```python
from build123d import *

# Parameters (mm, degrees)
SKETCH1_R               = 10
BOSS_EXTRUDE1_DEPTH     = 15
SKETCH2_R               = 12.5
BOSS_EXTRUDE2_DEPTH     = 20
SKETCH3_R               = 12
BOSS_EXTRUDE3_DEPTH     = 139.2
SKETCH4_R               = 4.5
CUT_EXTRUDE1_DEPTH      = 176.094660113
CUT_EXTRUDE2_DEPTH      = 176.094660212
CUT_EXTRUDE2_DEPTH_BACK = 176.094660212
SKETCH5_W               = 50.129657838
SKETCH5_H               = 19.874218845
LPATTERN1_COUNT         = 2
LPATTERN1_PITCH         = 25
CUT_EXTRUDE3_DEPTH      = 176.094660212
CUT_EXTRUDE3_DEPTH_BACK = 176.094660212
SKETCH6_W               = 35.820903931
SKETCH6_H               = 2.5


with BuildPart() as part:
    # Sketch1 → Boss-Extrude1 (new body)
    with BuildSketch(Plane.XY):
        Circle(SKETCH1_R)
    extrude(amount=BOSS_EXTRUDE1_DEPTH)

    # Sketch2 → Boss-Extrude2 (add)
    with BuildSketch(Plane.XY.offset(15)):
        Circle(SKETCH2_R)
    extrude(amount=BOSS_EXTRUDE2_DEPTH)

    # Sketch3 → Boss-Extrude3 (add)
    with BuildSketch(Plane.XY.offset(35)):
        Circle(SKETCH3_R)
    extrude(amount=BOSS_EXTRUDE3_DEPTH)

    # Sketch4 → Cut-Extrude1 (cut, symmetric)
    with BuildSketch(Plane(origin=(0, 0, 0), x_dir=(1, 0, 0), z_dir=(0, 1, 0))):
        with Locations(Location((0, -154.2, 0), (0, 0, 270))):
            Circle(SKETCH4_R)
    cut_extrude1 = extrude(amount=CUT_EXTRUDE1_DEPTH, both=True, mode=Mode.SUBTRACT)

    # Sketch5 → Cut-Extrude2 (cut, two sides: drawn at the far end of the back side and taken through both)
    with BuildSketch(Plane(origin=(0, 0, 0), x_dir=(1, 0, 0), z_dir=(0, 1, 0)).offset(-CUT_EXTRUDE2_DEPTH_BACK)):
        with Locations((-12.564828919, -5.062890578)):
            Rectangle(SKETCH5_W, SKETCH5_H)
    extrude(amount=CUT_EXTRUDE2_DEPTH + CUT_EXTRUDE2_DEPTH_BACK, mode=Mode.SUBTRACT)

    # LPattern1: Cut-Extrude1 ×2
    with Locations(*[(0, 0, -i * LPATTERN1_PITCH) for i in range(1, LPATTERN1_COUNT)]):
        add(cut_extrude1, mode=Mode.SUBTRACT)

    # Sketch6 → Cut-Extrude3 (cut, two sides: drawn at the far end of the back side and taken through both)
    with BuildSketch(Plane(origin=(0, 0, 0), x_dir=(1, 0, 0), z_dir=(0, 1, 0)).offset(-CUT_EXTRUDE3_DEPTH_BACK)):
        with Locations((-5.910451966, -172.95)):
            Rectangle(SKETCH6_W, SKETCH6_H)
    extrude(amount=CUT_EXTRUDE3_DEPTH + CUT_EXTRUDE3_DEPTH_BACK, mode=Mode.SUBTRACT)


solid = part.part
```
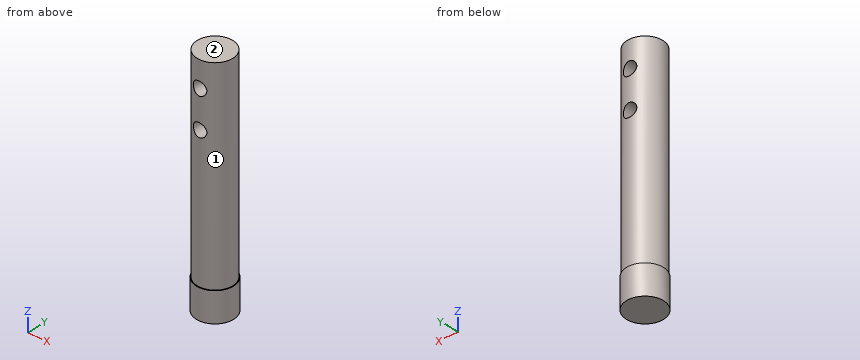
The listing builds one solid part. Answer for the finished solid, in the listing's coordinates (mm). Face numbers are marked on the shaded views. A direction names the side the tool comes from. Coordinates: 2 decimals unless noted, no trailing zeros. Write each loop counter-clockwise with the first axis right and the second up, starting at its lowest first coordinate (ties: lowest second). Pieces come first, ordered by that corner, then holes. Notation, with made-up numbers: M 29.5,-4 L 55.5,-4 A19 ccw 55.5,10 Z; hole C 5,5 d1. An arc over 180 degrees is marked long. Use a Markdown table: item, result. Add a question column.
1. Given P1, Ø12, axis at y = 7.5, z = 141, coming from the +X side; P2, Ø8, axis at x = 8, z = 54.5, coming from the +Y side; P3, Ø2, axis at x = 4, z = 143, coming from the -Y side; P4, Ø8, axis at x = 0, z = 129.2, coming from the +Y side, each flat-ended and moving along its own axis, determine where each tip first touches the part or whether it passes through.
2. Section C-C (z = 129.2) is taken. Give the vertices of the cut face in (x, y).
3. Straight lines are drawn through the part: line 1 along Z through (x, y) = (0, 4.5); line 2 along X through (y, z) = (-0.25, 129.2); line 3 along Z through (x, y) = (-3.5, 10.5). For each, find the intervals that lie inside material, in ascending order. Write a range as [from, to].
4. Which of the six approach directions +Z, -Z, +X, -X, +Y, -Y give full straight-line access (tool end or side, diameter ignored) to the marked faces 1 and 2?
5. Section B-B (x = 0) is taken. Give the vertices of the cut face in (y, z).
6. Section A-A (y = 0) is taken. Give the vertices of the cut face in (x, z), plus the area to 3 significant figures.
7. Section D-D (z = 111.5) is taken. Give the vertices of the cut face in (x, y).
Data:
| question | item | result |
|---|---|---|
| 1 | P1 | stops at x = 11.91 |
| 1 | P2 | stops at y = 11.31 |
| 1 | P3 | stops at y = -11.62 |
| 1 | P4 | passes through |
| 2 | outline | M -4.5,-11.12 L -4.5,11.12 A12 ccw Z; M 4.5,-11.12 A12 ccw 4.5,11.12 Z |
| 3 | line 1 | z = [15, 124.7], [133.7, 149.7], [158.7, 171.7] |
| 3 | line 2 | x = [-12, -4.5], [4.5, 12] |
| 3 | line 3 | z = [15, 126.37], [132.03, 151.37], [157.03, 171.7] |
| 4 | face 1 | +Z |
| 4 | face 2 | +Z, +X, -X, +Y, -Y |
| 5 | outline | M -12.5,15 L 12.5,15 L 12.5,35 L 12,35 L 12,124.7 L -12,124.7 L -12,35 L -12.5,35 Z; M -12,133.7 L 12,133.7 L 12,149.7 L -12,149.7 Z; M -12,158.7 L 12,158.7 L 12,171.7 L -12,171.7 Z |
| 6 | outline | M -12.5,15 L 12.5,15 L 12.5,35 L 12,35 L 12,171.7 L -12,171.7 L -12,35 L -12.5,35 Z; hole C 0,129.2 d9; hole C 0,154.2 d9 |
| 6 | area | 3,650 mm2 |
| 7 | outline | C 0,0 d24 |
